Check sheet for the modelled part. Datum: model origin and axes. Units: mm. Round coordinates to 2 decimals unless told otherwise and drop trailing zeros. Write each loop counter-clockwise with the first axis right and the second up, starting at its lowest first coordinate (ties: lowest second). Pieces come first, ordered by that corner, then holes. Notation, with made-up numbers: (78.5, 20.25) -> (97.5, 20.25) arc R18 cw to (97.5, 31.25) -> close; hole circle Ø5 at (63, -11.75). An arc over 180 degrees is marked (long way). Use one line per item in the form item = value. Start each with the question number.
```python
from build123d import *

# Parameters (mm, degrees)
SKETCH1_W           = 61.5
SKETCH1_H           = 203.2
BOSS_EXTRUDE1_DEPTH = 7.9375
SKETCH2_R           = 5.5
CUT_EXTRUDE1_DEPTH  = 16.875
SKETCH3_R           = 2.875
CUT_EXTRUDE2_DEPTH  = 16.875
LPATTERN1_COUNT     = 2
LPATTERN1_PITCH     = 32


with BuildPart() as part:
    # Sketch1 → Boss-Extrude1 (new body, symmetric)
    with BuildSketch(Plane.XY):
        Rectangle(SKETCH1_W, SKETCH1_H)
    extrude(amount=BOSS_EXTRUDE1_DEPTH, both=True)

    # Sketch2 → Cut-Extrude1 (cut, through all)
    with BuildSketch(Plane.XY.offset(7.9375)):
        with Locations((-21.25, 33.4)):
            Circle(SKETCH2_R)
        with Locations((-21.25, -1.6)):
            Circle(SKETCH2_R)
        with Locations((-21.25, -36.6)):
            Circle(SKETCH2_R)
        with Locations((-21.25, -71.6)):
            Circle(SKETCH2_R)
    extrude(amount=-CUT_EXTRUDE1_DEPTH, mode=Mode.SUBTRACT)

    # Sketch3 → Cut-Extrude2 (cut, through all)
    with BuildSketch(Plane.XY.offset(7.9375)):
        with Locations((-6.75, 80.85)):
            Circle(SKETCH3_R)
        with Locations((-6.75, 44.85)):
            Circle(SKETCH3_R)
        with Locations((-6.75, -6.75)):
            Circle(SKETCH3_R)
        with Locations((-6.75, -42.75)):
            Circle(SKETCH3_R)
    cut_extrude2 = extrude(amount=-CUT_EXTRUDE2_DEPTH, mode=Mode.SUBTRACT)

    # LPattern1: Cut-Extrude2 ×2
    with Locations(*[(i * LPATTERN1_PITCH, 0, 0) for i in range(1, LPATTERN1_COUNT)]):
        add(cut_extrude2, mode=Mode.SUBTRACT)


solid = part.part
```
1. Scan lines: probe 1 along Y at (x, z) = (25.25, -2.75) (3 decimals); probe 2 along Y at (x, z) = (-21.25, 2.5); probe 3 along X at (y, z) = (82, 3.25). Record each from-to range of solid material in increasing order.
2. Sectioned sample at C-C (z = -4). Give the number of separate pieces and of enclosed holes in the cut face, and give its area (3 significant figures).
3. Sectioned sample at B-B (x = -21.25). Enter the section's corners in (y, z).
4. Depth check by flat-ended pin: pin 1 (17.5 mm diameter, centred on x = -21.25, y = -36.6, fed in from +Z). Enter the tip coordinate at first touch or a pass-through.
5. Sectioned sample at A-A (y = -36.6). Enter the section's corners in (x, z).
6. Sectioned sample at D-D (x = -6.75). Enter the section's corners in (y, z) (1 decimal).
7. Mould release check, pull along Y, two halves, no side actions. Record for faces 1 (the face through (-30.75, -1, 0)), 2 (the face through (0, -101.6, 0)), 3 (the face through (-18.71, -76.48, 0.11)): +Y half, -Y half, draft (parallel to the pull), parting line (faces both ways), or undercut.
Returned:
q1.probe_1 = -101.6 to -45.625, -39.875 to -9.625, -3.875 to 41.975, 47.725 to 77.975, 83.725 to 101.6
q1.probe_2 = -101.6 to -77.1, -66.1 to -42.1, -31.1 to -7.1, 3.9 to 27.9, 38.9 to 101.6
q1.probe_3 = -30.75 to -9.38, -4.12 to 22.62, 27.88 to 30.75
q2.separate_pieces = 1
q2.enclosed_holes = 12
q2.area = 11,900 mm^2
q3.outline = (-101.6, -7.94) -> (-77.1, -7.94) -> (-77.1, 7.94) -> (-101.6, 7.94) -> close; (-66.1, -7.94) -> (-42.1, -7.94) -> (-42.1, 7.94) -> (-66.1, 7.94) -> close; (-31.1, -7.94) -> (-7.1, -7.94) -> (-7.1, 7.94) -> (-31.1, 7.94) -> close; (3.9, -7.94) -> (27.9, -7.94) -> (27.9, 7.94) -> (3.9, 7.94) -> close; (38.9, -7.94) -> (101.6, -7.94) -> (101.6, 7.94) -> (38.9, 7.94) -> close
q4.pin_1 = 7.94
q5.outline = (-30.75, -7.94) -> (-26.75, -7.94) -> (-26.75, 7.94) -> (-30.75, 7.94) -> close; (-15.75, -7.94) -> (30.75, -7.94) -> (30.75, 7.94) -> (-15.75, 7.94) -> close
q6.outline = (-101.6, -7.9) -> (-45.6, -7.9) -> (-45.6, 7.9) -> (-101.6, 7.9) -> close; (-39.9, -7.9) -> (-9.6, -7.9) -> (-9.6, 7.9) -> (-39.9, 7.9) -> close; (-3.9, -7.9) -> (42, -7.9) -> (42, 7.9) -> (-3.9, 7.9) -> close; (47.7, -7.9) -> (78, -7.9) -> (78, 7.9) -> (47.7, 7.9) -> close; (83.7, -7.9) -> (101.6, -7.9) -> (101.6, 7.9) -> (83.7, 7.9) -> close
q7.face_1 = draft
q7.face_2 = -Y half
q7.face_3 = undercut
